The listing builds one solid part. Answer for the finished solid, in the listing's coordinates (mm). A direction names the side the tool comes from. Round coordinates to 2 decimals unless told otherwise and drop trailing zeros. Loops run counter-clockwise (first coordinate to the right, second up) from the corner with the lowest first, then second, coordinate; pieces in that order, holes last. Notation, with made-up numbers: M 86.5,56.5 L 129.5,56.5 A19 cw 129.5,71.5 Z; hole C -2.75,-40 d4. An arc over 180 degrees is marked long. Answer as a JSON object with one key per item and string values.
```python
from build123d import *

# Parameters (mm, degrees)
CHAFL_N1_SIZE = 1.25


with BuildPart() as part:
    # Croquis1 → Revolución1 (revolve)
    with BuildSketch(Plane(origin=(0, 0, 0), x_dir=(0, 0, -1), z_dir=(1, 0, 0))):
        with BuildLine():
            Line((0, 0), (0, 85.55))
            Line((0, 85.55), (3.18, 85.55))
            Line((3.18, 85.55), (3.18, 17.954698654))
            ThreePointArc((3.18, 17.954698654), (9.896609701, 5.315721242), (24.13, 3.81))
            Line((24.13, 3.81), (26.67, 1.27))
            Line((26.67, 1.27), (26.67, 0))
            Line((26.67, 0), (0, 0))
        make_face()
    revolve(axis=Axis((0, 0, 0), (0, 1, 0)))

    # Chaflán1
    chafl_n1_edges = [part.edges().sort_by_distance(p)[0] for p in [
        (0, 85.55, 3.18),
    ]]
    chamfer(chafl_n1_edges, length=CHAFL_N1_SIZE)


solid = part.part
```
Item 1: Flat-ended cylindrical pins translate along their axes: P1, Ø6, axis at y = 16.5, z = -3.5, coming from the -X side; P2, Ø6, axis at x = 3.5, y = 34, coming from the -Z side. Find the tip coordinate at first contact, or state that the pin passes through.
Values follow:
{"P1": "x = -3.36", "P2": "z = -3.14"}
Item 2: The part is cut by section D-D (y = 6). Give the vertices of the cut face in (x, z).
Values follow:
{"outline": "C 0,0 d17.92"}
Item 3: The part is cut by section B-B (z = 0). Give the vertices of the cut face in (x, y).
Values follow:
{"outline": "M -26.67,0 L 26.67,0 L 26.67,1.27 L 24.13,3.81 A15.25 cw 3.18,17.95 L 3.18,84.3 L 1.93,85.55 L -1.93,85.55 L -3.18,84.3 L -3.18,17.95 A15.25 cw -24.13,3.81 L -26.67,1.27 Z"}
Item 4: Straight lines are drawn through the part: line 1 (Y direction, x = -24, z = 10); line 2 (Y direction, x = -19, z = -9.5); line 3 (Z direction, x = 2.5, y = 79). For each, find the intervals that lie inside material, in ascending order.
Values follow:
{"line 1": "0 to 1.94", "line 2": "0 to 2.97", "line 3": "-1.97 to 1.97"}
Item 5: The part is cut by section C-C (y = 69.5). Give the vertices of the cut face in (x, z), then the cut area to 3 significant figures.
Values follow:
{"outline": "C 0,0 d6.36", "area": "31.8 mm^2"}
Item 6: The part is cut by section A-A (x = 0). Give the vertices of the cut face in (y, z).
Values follow:
{"outline": "M 0,-26.67 L 1.27,-26.67 L 3.81,-24.13 A15.25 cw 17.95,-3.18 L 84.3,-3.18 L 85.55,-1.93 L 85.55,1.93 L 84.3,3.18 L 17.95,3.18 A15.25 cw 3.81,24.13 L 1.27,26.67 L 0,26.67 Z"}
Item 7: Which of the six approach directions +Z, -Z, +X, -X, +Y, -Y give full straight-line access (tool end or side, diameter ignored) to faces 1 (the face through (0, 85.55, 0)), 2 (the face through (3.1, 50.7, 0.7))?
Values follow:
{"face 1": "+Z, -Z, +X, -X, +Y", "face 2": "+Y"}
